Could you check a few things on this model? Use its own coordinates, in mm. Coordinates: 2 decimals unless noted, no trailing zeros. Write item = value, one per line.
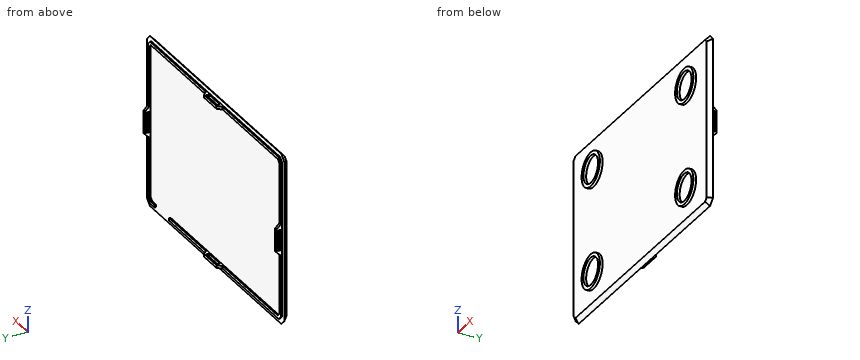
```python
from build123d import *

# Parameters (mm, degrees)
SKETCH_1_W          = 188
SKETCH_1_H          = 125
EXTRUDE_1_DEPTH     = 3
SKETCH_2_W          = 182
SKETCH_2_H          = 119
SKETCH_2_W_2        = 178
SKETCH_2_H_2        = 115
EXTRUDE_2_DEPTH     = 1
CUT_EXTRUDE_1_REACH = 156.042
SKETCH_4_W          = 20.2
SKETCH_4_H          = 1
SKETCH_5_W          = 15
SKETCH_5_H          = 2
SKETCH_5_W_2        = 2
SKETCH_5_H_2        = 15
EXTRUDE_3_DEPTH     = 3
CHAMFER_1_SIZE      = 4
CUT_EXTRUDE_2_REACH = 156.065
SKETCH_6_W          = 15
SKETCH_6_H          = 2
CUT_EXTRUDE_3_REACH = 197.313
SKETCH_7_W          = 15
SKETCH_7_H          = 2
SKETCH_8_R          = 12.5
EXTRUDE_4_DEPTH     = 2
SKETCH_9_R          = 10
CUT_EXTRUDE_4_DEPTH = 2
CHAMFER_2_SIZE      = 4
CHAMFER_3_SIZE      = 3
CHAMFER_4_SIZE      = 2
CHAMFER_5_SIZE      = 3


# Some blends are built 0.0001 mm under size
with BuildPart() as part:
    # 草图1 → 凸台-拉伸1 (new body)
    with BuildSketch(Plane(origin=(0, 0, 0), x_dir=(1, 0, 0), z_dir=(0, 1, 0))):
        Rectangle(SKETCH_1_W, SKETCH_1_H)
    extrude(amount=-EXTRUDE_1_DEPTH)

    # 草图2 → 凸台-拉伸2 (add)
    with BuildSketch(Plane(origin=(0, 0, 0), x_dir=(1, 0, 0), z_dir=(0, 1, 0))):
        Rectangle(SKETCH_2_W, SKETCH_2_H)
        Rectangle(SKETCH_2_W_2, SKETCH_2_H_2, mode=Mode.SUBTRACT)
    extrude(amount=EXTRUDE_2_DEPTH)

    # 草图4 → 切除-拉伸1 (cut, up to next)
    with BuildSketch(Plane(origin=(0, 0, -59.5), x_dir=(-1, 0, 0), z_dir=(0, 0, -1)), mode=Mode.PRIVATE) as cut_extrude_1_sk1:
        with Locations((-71.9, 0.5)):
            Rectangle(SKETCH_4_W, SKETCH_4_H)
    cut_extrude_1_tool1 = extrude(cut_extrude_1_sk1.sketch, amount=-CUT_EXTRUDE_1_REACH, mode=Mode.PRIVATE) & part.part
    add(cut_extrude_1_tool1.solids().sort_by_distance((71.9, 0.5, -59.5))[0], mode=Mode.SUBTRACT)

    # 草图5 → 凸台-拉伸3 (add)
    with BuildSketch(Plane(origin=(0, 1, 0), x_dir=(1, 0, 0), z_dir=(0, 1, 0))):
        with Locations((0, -58.5)):
            Rectangle(SKETCH_5_W, SKETCH_5_H)
        with Locations((90, 0)):
            Rectangle(SKETCH_5_W_2, SKETCH_5_H_2)
        with Locations((0, 58.5)):
            Rectangle(SKETCH_5_W, SKETCH_5_H)
        with Locations((-90, 0)):
            Rectangle(SKETCH_5_W_2, SKETCH_5_H_2)
    extrude(amount=EXTRUDE_3_DEPTH)

    # 倒角1
    # the kernel refuses this chamfer: 4 mm, written as the material it adds along each edge
    with BuildSketch(Plane(origin=(-89, 1, -7.5), x_dir=(0, -0.027495876610586372, -0.9996219169112968), z_dir=(-1, 0, 0))) as chamfer_1_piece_1_section:
        Polygon((CHAMFER_1_SIZE * 0.999621916911, -CHAMFER_1_SIZE * 0.0274958766106), (-CHAMFER_1_SIZE * 0.0274958766106, -CHAMFER_1_SIZE * 0.999621916911), (0, 0), align=None)
    chamfer_1_piece_1 = extrude(amount=2, mode=Mode.PRIVATE)
    chamfer_1_piece_1 = split(chamfer_1_piece_1, bisect_by=Plane(origin=(-90, 4, -8.907836441), z_dir=(0, -1, 0)), keep=Keep.TOP, mode=Mode.PRIVATE)
    add(chamfer_1_piece_1)
    with BuildSketch(Plane(origin=(-91, 1, 7.5), x_dir=(0, -0.027495876610586382, 0.9996219169112968), z_dir=(1, 0, 0))) as chamfer_1_piece_2_section:
        Polygon((CHAMFER_1_SIZE * 0.999621916911, -CHAMFER_1_SIZE * 0.0274958766106), (-CHAMFER_1_SIZE * 0.0274958766106, -CHAMFER_1_SIZE * 0.999621916911), (0, 0), align=None)
    chamfer_1_piece_2 = extrude(amount=2, mode=Mode.PRIVATE)
    chamfer_1_piece_2 = split(chamfer_1_piece_2, bisect_by=Plane(origin=(-90, 4, 8.907836441), z_dir=(0, -1, 0)), keep=Keep.TOP, mode=Mode.PRIVATE)
    add(chamfer_1_piece_2)
    with BuildSketch(Plane(origin=(-7.5, 1, 57.5), x_dir=(-0.9996219169112968, -0.027495876610586382, 0), z_dir=(0, 0, 1))) as chamfer_1_piece_3_section:
        Polygon((CHAMFER_1_SIZE * 0.999621916911, -CHAMFER_1_SIZE * 0.0274958766106), (-CHAMFER_1_SIZE * 0.0274958766106, -CHAMFER_1_SIZE * 0.999621916911), (0, 0), align=None)
    chamfer_1_piece_3 = extrude(amount=2, mode=Mode.PRIVATE)
    chamfer_1_piece_3 = split(chamfer_1_piece_3, bisect_by=Plane(origin=(-8.907836441, 4, 58.5), z_dir=(0, -1, 0)), keep=Keep.TOP, mode=Mode.PRIVATE)
    add(chamfer_1_piece_3)
    with BuildSketch(Plane(origin=(7.5, 1, 59.5), x_dir=(0.9996219169112968, -0.02749587661058638, 0), z_dir=(0, 0, -1))) as chamfer_1_piece_4_section:
        Polygon((CHAMFER_1_SIZE * 0.999621916911, -CHAMFER_1_SIZE * 0.0274958766106), (-CHAMFER_1_SIZE * 0.0274958766106, -CHAMFER_1_SIZE * 0.999621916911), (0, 0), align=None)
    chamfer_1_piece_4 = extrude(amount=2, mode=Mode.PRIVATE)
    chamfer_1_piece_4 = split(chamfer_1_piece_4, bisect_by=Plane(origin=(8.907836441, 4, 58.5), z_dir=(0, -1, 0)), keep=Keep.TOP, mode=Mode.PRIVATE)
    add(chamfer_1_piece_4)
    with BuildSketch(Plane(origin=(89, 1, 7.5), x_dir=(0, -0.027495876610586372, 0.9996219169112968), z_dir=(1, 0, 0))) as chamfer_1_piece_5_section:
        Polygon((CHAMFER_1_SIZE * 0.999621916911, -CHAMFER_1_SIZE * 0.0274958766106), (-CHAMFER_1_SIZE * 0.0274958766106, -CHAMFER_1_SIZE * 0.999621916911), (0, 0), align=None)
    chamfer_1_piece_5 = extrude(amount=2, mode=Mode.PRIVATE)
    chamfer_1_piece_5 = split(chamfer_1_piece_5, bisect_by=Plane(origin=(90, 4, 8.907836441), z_dir=(0, -1, 0)), keep=Keep.TOP, mode=Mode.PRIVATE)
    add(chamfer_1_piece_5)
    with BuildSketch(Plane(origin=(91, 1, -7.5), x_dir=(0, -0.02749587661058638, -0.9996219169112968), z_dir=(-1, 0, 0))) as chamfer_1_piece_6_section:
        Polygon((CHAMFER_1_SIZE * 0.999621916911, -CHAMFER_1_SIZE * 0.0274958766106), (-CHAMFER_1_SIZE * 0.0274958766106, -CHAMFER_1_SIZE * 0.999621916911), (0, 0), align=None)
    chamfer_1_piece_6 = extrude(amount=2, mode=Mode.PRIVATE)
    chamfer_1_piece_6 = split(chamfer_1_piece_6, bisect_by=Plane(origin=(90, 4, -8.907836441), z_dir=(0, -1, 0)), keep=Keep.TOP, mode=Mode.PRIVATE)
    add(chamfer_1_piece_6)
    with BuildSketch(Plane(origin=(-7.5, 1, -59.5), x_dir=(-0.9996219169112968, -0.02749587661058638, 0), z_dir=(0, 0, 1))) as chamfer_1_piece_7_section:
        Polygon((CHAMFER_1_SIZE * 0.999621916911, -CHAMFER_1_SIZE * 0.0274958766106), (-CHAMFER_1_SIZE * 0.0274958766106, -CHAMFER_1_SIZE * 0.999621916911), (0, 0), align=None)
    chamfer_1_piece_7 = extrude(amount=2, mode=Mode.PRIVATE)
    chamfer_1_piece_7 = split(chamfer_1_piece_7, bisect_by=Plane(origin=(-8.907836441, 4, -58.5), z_dir=(0, -1, 0)), keep=Keep.TOP, mode=Mode.PRIVATE)
    add(chamfer_1_piece_7)
    with BuildSketch(Plane(origin=(7.5, 1, -57.5), x_dir=(0.9996219169112968, -0.027495876610586372, 0), z_dir=(0, 0, -1))) as chamfer_1_piece_8_section:
        Polygon((CHAMFER_1_SIZE * 0.999621916911, -CHAMFER_1_SIZE * 0.0274958766106), (-CHAMFER_1_SIZE * 0.0274958766106, -CHAMFER_1_SIZE * 0.999621916911), (0, 0), align=None)
    chamfer_1_piece_8 = extrude(amount=2, mode=Mode.PRIVATE)
    chamfer_1_piece_8 = split(chamfer_1_piece_8, bisect_by=Plane(origin=(8.907836441, 4, -58.5), z_dir=(0, -1, 0)), keep=Keep.TOP, mode=Mode.PRIVATE)
    add(chamfer_1_piece_8)

    # 切除-拉伸2: up to this face of the body (flat: up to its plane)
    cut_extrude_2_end = Plane(part.part.faces().sort_by_distance((0, 0.977272727, 59.5))[0])
    # 草图6 → 切除-拉伸2 (cut, up to the picked face)
    with BuildSketch(Plane(origin=(0, 0, -59.5), x_dir=(-1, 0, 0), z_dir=(0, 0, -1)), mode=Mode.PRIVATE) as cut_extrude_2_sk1:
        with Locations((0, 2)):
            Rectangle(SKETCH_6_W, SKETCH_6_H)
    cut_extrude_2_tool1 = split(extrude(cut_extrude_2_sk1.sketch, amount=-CUT_EXTRUDE_2_REACH, mode=Mode.PRIVATE), bisect_by=cut_extrude_2_end, keep=Keep.BOTH, mode=Mode.PRIVATE)
    add(cut_extrude_2_tool1.solids().sort_by(Axis((0, 2, -59.5), (0, 0, 1)))[0], mode=Mode.SUBTRACT)

    # 切除-拉伸3: up to this face of the body (flat: up to its plane)
    cut_extrude_3_end = Plane(part.part.faces().sort_by_distance((91, 1.145251397, 0))[0])
    # 草图7 → 切除-拉伸3 (cut, up to the picked face)
    with BuildSketch(Plane.ZY.offset(91), mode=Mode.PRIVATE) as cut_extrude_3_sk1:
        with Locations((0, 2)):
            Rectangle(SKETCH_7_W, SKETCH_7_H)
    cut_extrude_3_tool1 = split(extrude(cut_extrude_3_sk1.sketch, amount=-CUT_EXTRUDE_3_REACH, mode=Mode.PRIVATE), bisect_by=cut_extrude_3_end, keep=Keep.BOTH, mode=Mode.PRIVATE)
    add(cut_extrude_3_tool1.solids().sort_by(Axis((-91, 2, 0), (1, 0, 0)))[0], mode=Mode.SUBTRACT)

    # 草图8 → 凸台-拉伸4 (add)
    with BuildSketch(Plane.XZ.offset(3)):
        with Locations(Location((-64, 37.5, 0), (0, 0, 90))):
            Circle(SKETCH_8_R)
        with Locations(Location((-64, -37.5, 0), (0, 0, 90))):
            Circle(SKETCH_8_R)
        with Locations(Location((64, 37.5, 0), (0, 0, 90))):
            Circle(SKETCH_8_R)
        with Locations(Location((64, -37.5, 0), (0, 0, 90))):
            Circle(SKETCH_8_R)
    extrude(amount=EXTRUDE_4_DEPTH)

    # 草图9 → 切除-拉伸4 (cut)
    with BuildSketch(Plane.XZ.offset(3)):
        with Locations(Location((-64, 37.5, 0), (0, 0, 270))):
            Circle(SKETCH_9_R)
        with Locations(Location((-64, -37.5, 0), (0, 0, 90))):
            Circle(SKETCH_9_R)
        with Locations(Location((64, 37.5, 0), (0, 0, 90))):
            Circle(SKETCH_9_R)
        with Locations(Location((64, -37.5, 0), (0, 0, 270))):
            Circle(SKETCH_9_R)
    extrude(amount=CUT_EXTRUDE_4_DEPTH, mode=Mode.SUBTRACT)

    # 倒角2
    chamfer_2_edges = [part.edges().sort_by_distance(p)[0] for p in [
        (-94, -1.5, -62.5),
        (94, -1.5, -62.5),
        (94, -1.5, 62.5),
        (-94, -1.5, 62.5),
    ]]
    chamfer(chamfer_2_edges, length=CHAMFER_2_SIZE)

    # 倒角3
    chamfer_3_edges = [part.edges().sort_by_distance(p)[0] for p in [
        (92, -3, -60.5),
        (0, -3, -62.5),
        (-92, -3, -60.5),
        (-94, -3, 0),
        (-92, -3, 60.5),
        (0, -3, 62.5),
        (92, -3, 60.5),
        (94, -3, 0),
    ]]
    chamfer(chamfer_3_edges, length=CHAMFER_3_SIZE - 0.0001)  # a hair under: the kernel refuses the full size

    # 倒角4
    chamfer_4_edges = [part.edges().sort_by_distance(p)[0] for p in [
        (-89, 0.5, 57.5),
        (89, 0.5, 57.5),
        (89, 0.5, -57.5),
        (-89, 0.5, -57.5),
    ]]
    chamfer(chamfer_4_edges, length=CHAMFER_4_SIZE)

    # 倒角5
    chamfer_5_edges = [part.edges().sort_by_distance(p)[0] for p in [
        (-91, 0.5, -59.5),
        (-91, 0.5, 59.5),
        (91, 0.5, 59.5),
        (91, 0.5, -59.5),
    ]]
    chamfer(chamfer_5_edges, length=CHAMFER_5_SIZE)


solid = part.part
```
Item 1: If I drill on line 1 along X through (y, z) = (-4.55, 37.5); line 2 along X through (y, z) = (0.5, 37); line 3 along Y through (x, z) = (-18.5, -48.5), over which ranges is the centre line in solid material (lowest first)?
Numbers:
line_1 = -76.5 to -74, -54 to -51.5, 51.5 to 54, 74 to 76.5
line_2 = -91 to -89, 89 to 91
line_3 = -3 to 0
Item 2: Imagine slicing it at A-A (z = -0.5). State how many separate pieces and enclosed holes the cut face has, and give its area (3 significant figures).
Numbers:
separate_pieces = 3
enclosed_holes = 0
area = 563 mm²
Item 3: I'm going to push flat-ended pins straight in: P1, Ø4, axis at x = -19, z = 5.5, coming from the -Y side; P2, Ø12, axis at x = 64, z = -37.5, coming from the +Y side; P3, Ø3, axis at x = -38, y = -4, coming from the -Z side. Where does each tip first touch, or does it pass through?
Numbers:
P1 = -3
P2 = 0
P3 = -60
